```python
from build123d import *

# Parameters (mm, degrees)
SALIENTE_EXTRUIR1_DEPTH = 50
CORTAR_EXTRUIR1_REACH   = 10
CROQUIS3_R              = 1.6
CROQUIS6_R              = 1.9
CORTAR_EXTRUIR3_DEPTH   = 10


with BuildPart() as part:
    # Croquis1 → Saliente-Extruir1 (new body)
    with BuildSketch(Plane.XY):
        Polygon((45.761533754, 80.324875029), (73.190105182, 80.324875029), (69.761533754, 72.324875029), (45.761533754, 72.324875029), align=None)
    extrude(amount=SALIENTE_EXTRUIR1_DEPTH)

    # Croquis3 → Cortar-Extruir1 (cut, up to next)
    with BuildSketch(Plane.XZ.offset(-72.324875029), mode=Mode.PRIVATE) as cortar_extruir1_sk1:
        with Locations((63.761533754, 35)):
            Circle(CROQUIS3_R)
    cortar_extruir1_tool1 = extrude(cortar_extruir1_sk1.sketch, amount=-CORTAR_EXTRUIR1_REACH, mode=Mode.PRIVATE) & part.part
    add(cortar_extruir1_tool1.solids().sort_by_distance((63.761534, 72.324875, 35))[0], mode=Mode.SUBTRACT)
    # Croquis3 → Cortar-Extruir1 (cut, up to next)
    with BuildSketch(Plane.XZ.offset(-72.324875029), mode=Mode.PRIVATE) as cortar_extruir1_sk2:
        with Locations((57.761533754, 20)):
            Circle(CROQUIS3_R)
    cortar_extruir1_tool2 = extrude(cortar_extruir1_sk2.sketch, amount=-CORTAR_EXTRUIR1_REACH, mode=Mode.PRIVATE) & part.part
    add(cortar_extruir1_tool2.solids().sort_by_distance((57.761534, 72.324875, 20))[0], mode=Mode.SUBTRACT)
    # Croquis3 → Cortar-Extruir1 (cut, up to next)
    with BuildSketch(Plane.XZ.offset(-72.324875029), mode=Mode.PRIVATE) as cortar_extruir1_sk3:
        with Locations((51.761533754, 35)):
            Circle(CROQUIS3_R)
    cortar_extruir1_tool3 = extrude(cortar_extruir1_sk3.sketch, amount=-CORTAR_EXTRUIR1_REACH, mode=Mode.PRIVATE) & part.part
    add(cortar_extruir1_tool3.solids().sort_by_distance((51.761534, 72.324875, 35))[0], mode=Mode.SUBTRACT)

    # Croquis6 → Cortar-Extruir3 (cut)
    with BuildSketch(Plane(origin=(0, 0, 0), x_dir=(-1, 0, 0), z_dir=(0, 0, -1))):
        with Locations((-66.332962325, 76.324875029)):
            Circle(CROQUIS6_R)
        with Locations((-52.618676611, 76.324875029)):
            Circle(CROQUIS6_R)
    extrude(amount=-CORTAR_EXTRUIR3_DEPTH, mode=Mode.SUBTRACT)


solid = part.part
```
Here's how the part is built. I have some questions about the finished solid (model axes, mm). A direction names the side the tool comes from. Coordinates: 2 decimals unless noted, no trailing zeros. Write each loop counter-clockwise with the first axis right and the second up, starting at its lowest first coordinate (ties: lowest second). Pieces come first, ordered by that corner, then holes. Notation, with made-up numbers: (76, -38) -> (118, -38) arc R25 ccw to (118, -18) -> close; hole circle Ø5 at (19.25, 58). An arc over 180 degrees is marked (long way). Use a Markdown table: item, result. Add a question column.
(1) For faces 4 (the flat face through (53, 76, 10)), 5 (the cylindrical face through (53.24, 76.27, 34.39)), which set-ups out of +Z, -Z, +X, -X, +Y, -Y let a thin tool reach every point of the face, with its end or its side?
(2) If we section it at D-D, the plane x = 62.75: Write out the boundary of the cut face in (y, z), and give its area (3 significant figures).
(3) Please list where these lines run through material, in increasing order: line 1 (X direction, y = 77.25, z = 9); line 2 (Z direction, x = 64.75, y = 79); line 3 (Z direction, x = 64, y = 76.25).
(4) I'm going to push flat-ended pins straight in: P1, Ø3, axis at x = 51.76, z = 35, coming from the +Y side; P2, Ø3.5, axis at x = 66.33, y = 76.32, coming from the -Z side; P3, Ø4, axis at y = 73.5, z = 23, coming from the +X side. Where does each tip first touch, or does it pass through?
(5) If we section it at C-C, the plane y = 77.5: Write out the boundary of the cut face in (x, z), and give its area (3 significant figures).
(6) If we section it at A-A, the plane z = 35: Write out the boundary of the cut face in (x, y), and give its area (3 significant figures).
(7) We'd pull the mould along X, two halves only. Please class faces 1 (the flat face through (71.5, 76.38, 24.65)), 2 (the flat face through (66, 76, 10)), 3 (the flat face through (60, 76, 50)): +X half, -X half, draft (parallel to the pull), parting line (faces both ways), or undercut.
(8) If we section it at B-B, the plane z = 20: Write out the boundary of the cut face in (x, y), and give its area (3 significant figures).
Outcome:
| question | item | result |
|---|---|---|
| 1 | face 4 | -Z |
| 1 | face 5 | +Y, -Y |
| 2 | outline | (72.32, 0) -> (80.32, 0) -> (80.32, 33.76) -> (72.32, 33.76) -> close; (72.32, 36.24) -> (80.32, 36.24) -> (80.32, 50) -> (72.32, 50) -> close |
| 2 | area | 380 mm^2 |
| 3 | line 1 | x = 45.76 to 50.96, 54.28 to 64.67, 67.99 to 71.87 |
| 3 | line 2 | z = 0 to 33.74, 36.26 to 50 |
| 3 | line 3 | z = 0 to 33.42, 36.58 to 50 |
| 4 | P1 | passes through |
| 4 | P2 | stops at z = 10 |
| 4 | P3 | stops at x = 71.12 |
| 5 | outline | (45.76, 0) -> (51.13, 0) -> (51.13, 10) -> (54.11, 10) -> (54.11, 0) -> (64.84, 0) -> (64.84, 10) -> (67.83, 10) -> (67.83, 0) -> (71.98, 0) -> (71.98, 50) -> (45.76, 50) -> close; hole circle Ø3.2 at (51.76, 35); hole circle Ø3.2 at (57.76, 20); hole circle Ø3.2 at (63.76, 35) |
| 5 | area | 1,230 mm^2 |
| 6 | outline | (45.76, 72.32) -> (50.16, 72.32) -> (50.16, 80.32) -> (45.76, 80.32) -> close; (53.36, 72.32) -> (62.16, 72.32) -> (62.16, 80.32) -> (53.36, 80.32) -> close; (65.36, 72.32) -> (69.76, 72.32) -> (73.19, 80.32) -> (65.36, 80.32) -> close |
| 6 | area | 155 mm^2 |
| 7 | face 1 | +X half |
| 7 | face 2 | undercut |
| 7 | face 3 | draft |
| 8 | outline | (45.76, 72.32) -> (56.16, 72.32) -> (56.16, 80.32) -> (45.76, 80.32) -> close; (59.36, 72.32) -> (69.76, 72.32) -> (73.19, 80.32) -> (59.36, 80.32) -> close |
| 8 | area | 180 mm^2 |
